Could you check a few things on this drawing? It's one solid part, dimensions in mm from its lowest x, y, z. A direction names the side the tool comes from. Coordinates: 2 decimals unless noted, no trailing zeros. Order: outer loops, then holes, each group sorted by start corner. A loop starts at its lowest first (then second) coordinate and runs counter-clockwise, first axis right, second up. Notation, with made-up numbers: (21, -24) -> (49, -24) arc R29 cw to (49, 13) -> close; hole circle Ø6 at (37.25, 81.5). An arc over 180 degrees is marked (long way). Use a Markdown table: item, result. Add a question column.
1. For the marked faces 4, 5, 6 and 7, which set-ups out of +Z, -Z, +X, -X, +Y, -Y let a thin tool reach every point of the face, with its end or its side?
2. We'd pull the mould along X, two halves only. Please class the marked faces 1, 2 and 3: pulls with the +X half, pulls with the -X half, needs draft (parallel to the pull), parting line crosses it, or undercut.
3. Suppose I cut it at C-C, the plane x = 60. List the corners of the cut face in (y, z) for me.
4. For pin 1 Ø4.5 at (x, y) = (9, 10.5) entering from -Z; pin 2 Ø5 at (x, z) = (8.5, 29.5) entering from -Y; pin 3 Ø12 at (x, y) = (62.5, 8) entering from +Z; pin 4 Ø4 at (x, z) = (29.5, 30.5) entering from -Y, each with a flat end and sliding along its axis, tell me the tip position at first contact or that it passes through.
5. Suppose I cut it at D-D, the plane z = 12. List the corners of the cut face in (x, y) for me, then the cut area to 3 significant figures.
6. If I drill on line 1 along X through (y, z) = (8, 33); line 2 along Z through (x, y) = (57, 18.5); line 3 along Y through (x, z) = (58.5, 7), over which ranges is the centre line in solid material (lowest first)? Write a range as from..to.
7. Suppose I cut it at B-B, the plane z = 34.5. List the corners of the cut face in (x, y) for me.
8. Suppose I cut it at A-A, the plane y = 13. List the corners of the cut face in (x, z) for me.
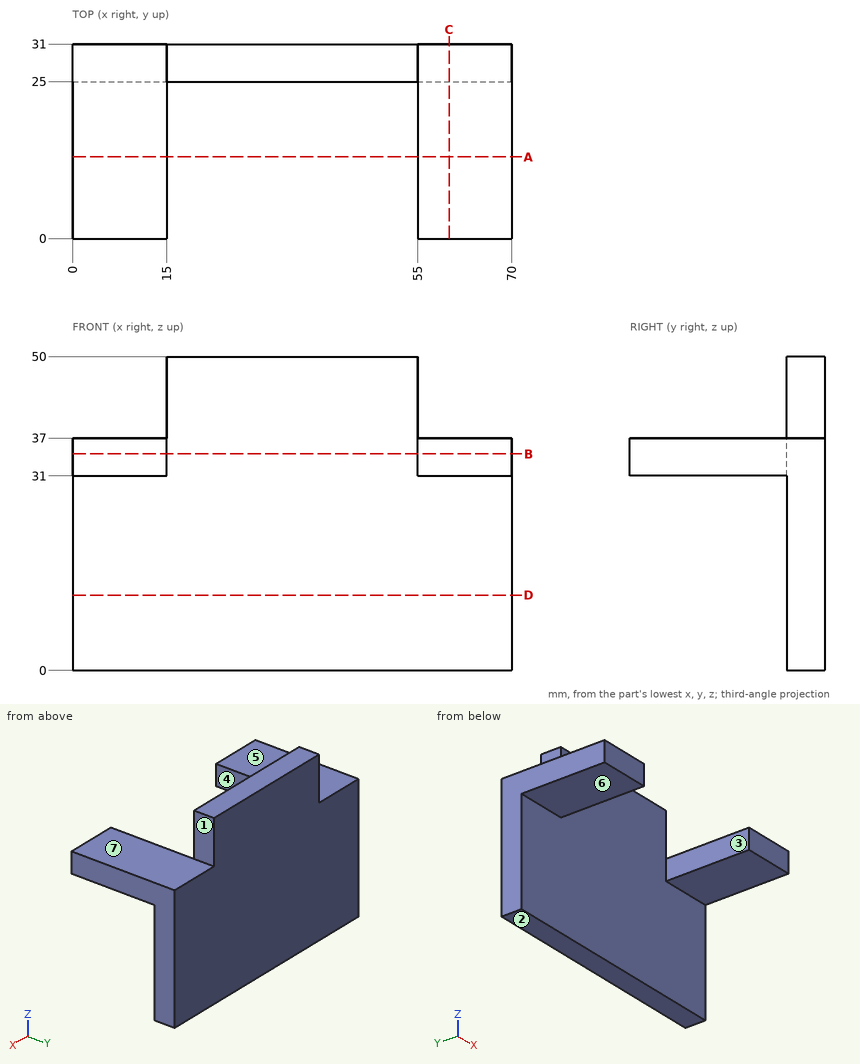
Worked out:
| question | item | result |
|---|---|---|
| 1 | face 4 | +Z, -Z, -Y |
| 1 | face 5 | +Z, -X, +Y, -Y |
| 1 | face 6 | -Z, +X, -X, -Y |
| 1 | face 7 | +Z, +X, +Y, -Y |
| 2 | face 1 | pulls with the +X half |
| 2 | face 2 | needs draft |
| 2 | face 3 | undercut |
| 3 | outline | (0, 31) -> (25, 31) -> (25, 0) -> (31, 0) -> (31, 37) -> (0, 37) -> close |
| 4 | pin 1 | stops at z = 31 |
| 4 | pin 2 | stops at y = 0 |
| 4 | pin 3 | stops at z = 37 |
| 4 | pin 4 | stops at y = 25 |
| 5 | outline | (0, 25) -> (70, 25) -> (70, 31) -> (0, 31) -> close |
| 5 | area | 420 mm² |
| 6 | line 1 | x = 0..15, 55..70 |
| 6 | line 2 | z = 31..37 |
| 6 | line 3 | y = 25..31 |
| 7 | outline | (0, 0) -> (15, 0) -> (15, 25) -> (55, 25) -> (55, 0) -> (70, 0) -> (70, 31) -> (0, 31) -> close |
| 8 | outline | (0, 31) -> (15, 31) -> (15, 37) -> (0, 37) -> close; (55, 31) -> (70, 31) -> (70, 37) -> (55, 37) -> close |
